Work out the finished part from the listing and answer in its coordinate system (mm). Face numbers are marked on the shaded views. A direction names the side the tool comes from. Round coordinates to 2 decimals unless told otherwise and drop trailing zeros. Write each loop counter-clockwise with the first axis right and the second up, starting at its lowest first coordinate (ties: lowest second). Pieces come first, ordered by that corner, then holes. Notation, with made-up numbers: M 89.25,-16 L 126.25,-16 A32 cw 126.25,23 Z; hole C 26.25,19 d1. An arc over 180 degrees is marked long. One line per item, written item: value. Start each with the question number.
Q1. Find section A-A (y = 0). Write down the section's boundary in (x, z), and give its area (3 significant figures).
Q2. Find section B-B (x = 1). Write down the section's boundary in (y, z), and give its area (3 significant figures).
Q3. Given pin 1 Ø1 at (x, y) = (0, -16.5) entering from +Z; pin 2 Ø2.5 at (x, z) = (-18.5, 1.5) entering from -Y; pin 3 Ø5 at (x, y) = (-19.5, -1) entering from +Z, each flat-ended and moving along its own axis, determine where each tip first touches the part or whether it passes through.
Q4. The mould has two halves that part along X. Classify the marked faces 1, 2 and 3: released by +X, released by -X, zero draft, split by the parting line, or undercut.
Q5. Consider probe 1 along X at (y, z) = (12, 6.75); probe 2 along X at (y, z) = (12, 8.5); probe 3 along Y at (x, z) = (-9, 13.75). Determine where each line is inside the solid, lowest interval first.
Q6. Find section C-C (z = 6). Write down the section's boundary in (x, y).
Q7. Find section D-D (z = 11.25). Write down the section's boundary in (x, y), and give its area (3 significant figures).
Q8. A tool of negligible diameter and unlimited length cuts with its end or side. For the marked faces 4, 5 and 6, from which of +Z, -Z, +X, -X, +Y, -Y can it reach the whole face along a straight path? Write none if from no direction.
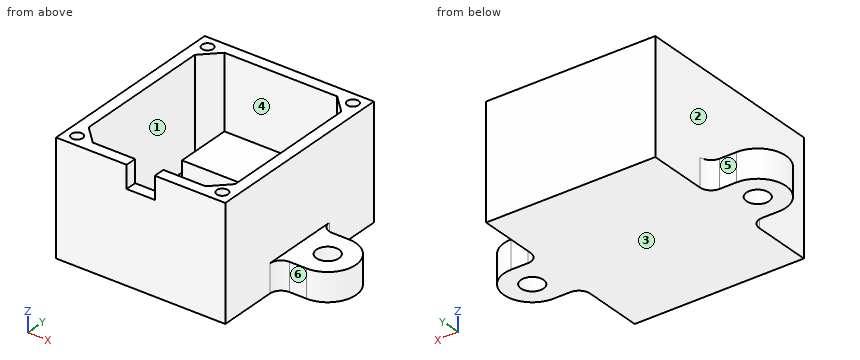
from build123d import *

# Parameters (mm, degrees)
ESQUISSE1_W             = 30
ESQUISSE1_H             = 35
BOSS_EXTRU_1_DEPTH      = 20
ENL_V_MAT_EXTRU_1_DEPTH = 18
BOSS_EXTRU_2_DEPTH      = 5
ENL_V_MAT_EXTRU_2_REACH = 7
ESQUISSE4_R             = 2
ESQUISSE5_W             = 20
ESQUISSE5_H             = 10
BOSS_EXTRU_3_DEPTH      = 5
ENL_V_MAT_EXTRU_3_REACH = 37
ESQUISSE6_W             = 5
ESQUISSE6_H             = 4
CONG_1_R                = 2
ESQUISSE7_R             = 1
ENL_V_MAT_EXTRU_4_DEPTH = 10


with BuildPart() as part:
    # Esquisse1 → Boss.-Extru.1 (new body)
    with BuildSketch(Plane.XY):
        Rectangle(ESQUISSE1_W, ESQUISSE1_H)
    extrude(amount=BOSS_EXTRU_1_DEPTH)

    # Esquisse2 → Enlèv. mat.-Extru.1 (cut)
    with BuildSketch(Plane.XY.offset(20)):
        Polygon((-10, 15.5), (10, 15.5), (13, 12.5), (13, -12.5), (10, -15.5), (-10, -15.5), (-13, -12.5), (-13, 12.5), align=None)
    extrude(amount=-ENL_V_MAT_EXTRU_1_DEPTH, mode=Mode.SUBTRACT)

    # Esquisse3 → Boss.-Extru.2 (add)
    with BuildSketch(Plane(origin=(0, 0, 0), x_dir=(-1, 0, 0), z_dir=(0, 0, -1))):
        with BuildLine():
            Line((-15, 5), (-20, 5))
            ThreePointArc((-20, 5), (-25, 0), (-20, -5))
            Line((-20, -5), (-15, -5))
            Line((-15, -5), (-15, 5))
        make_face()
        with BuildLine():
            Line((15, 5), (15, -5))
            Line((15, -5), (20, -5))
            ThreePointArc((20, -5), (25, 0), (20, 5))
            Line((20, 5), (15, 5))
        make_face()
    extrude(amount=-BOSS_EXTRU_2_DEPTH)

    # Esquisse4 → Enlèv. mat.-Extru.2 (cut, up to next)
    with BuildSketch(Plane.XY.offset(5), mode=Mode.PRIVATE) as enl_v_mat_extru_2_sk1:
        with Locations((-20, 0)):
            Circle(ESQUISSE4_R)
    enl_v_mat_extru_2_tool1 = extrude(enl_v_mat_extru_2_sk1.sketch, amount=-ENL_V_MAT_EXTRU_2_REACH, mode=Mode.PRIVATE) & part.part
    add(enl_v_mat_extru_2_tool1.solids().sort_by_distance((-20, 0, 5))[0], mode=Mode.SUBTRACT)
    # Esquisse4 → Enlèv. mat.-Extru.2 (cut, up to next)
    with BuildSketch(Plane.XY.offset(5), mode=Mode.PRIVATE) as enl_v_mat_extru_2_sk2:
        with Locations((20, 0)):
            Circle(ESQUISSE4_R)
    enl_v_mat_extru_2_tool2 = extrude(enl_v_mat_extru_2_sk2.sketch, amount=-ENL_V_MAT_EXTRU_2_REACH, mode=Mode.PRIVATE) & part.part
    add(enl_v_mat_extru_2_tool2.solids().sort_by_distance((20, 0, 5))[0], mode=Mode.SUBTRACT)

    # Esquisse5 → Boss.-Extru.3 (add)
    with BuildSketch(Plane.XY.offset(2)):
        with Locations((0, 10.5)):
            Rectangle(ESQUISSE5_W, ESQUISSE5_H)
    extrude(amount=BOSS_EXTRU_3_DEPTH)

    # Esquisse6 → Enlèv. mat.-Extru.3 (cut, up to next)
    with BuildSketch(Plane.XZ.offset(17.5), mode=Mode.PRIVATE) as enl_v_mat_extru_3_sk1:
        with Locations((0, 18)):
            Rectangle(ESQUISSE6_W, ESQUISSE6_H)
    enl_v_mat_extru_3_tool1 = extrude(enl_v_mat_extru_3_sk1.sketch, amount=-ENL_V_MAT_EXTRU_3_REACH, mode=Mode.PRIVATE) & part.part
    add(enl_v_mat_extru_3_tool1.solids().sort_by_distance((0, -17.5, 18))[0], mode=Mode.SUBTRACT)

    # Congé1
    cong_1_edges = [part.edges().sort_by_distance(p)[0] for p in [
        (15, -5, 2.5),
        (15, 5, 2.5),
        (-15, 5, 2.5),
        (-15, -5, 2.5),
    ]]
    fillet(cong_1_edges, radius=CONG_1_R)

    # Esquisse7 → Enlèv. mat.-Extru.4 (cut)
    with BuildSketch(Plane.XY.offset(20)):
        with Locations((-12.878679656, 15.378679656)):
            Circle(ESQUISSE7_R)
        with Locations((-12.878679656, -15.378679656)):
            Circle(ESQUISSE7_R)
        with Locations((12.878679656, -15.378679656)):
            Circle(ESQUISSE7_R)
        with Locations((12.878679656, 15.378679656)):
            Circle(ESQUISSE7_R)
    extrude(amount=-ENL_V_MAT_EXTRU_4_DEPTH, mode=Mode.SUBTRACT)


solid = part.part
The answers:
1. outline: M -25,0 L -22,0 L -22,5 L -25,5 Z; M -18,0 L 18,0 L 18,5 L 15,5 L 15,20 L 13,20 L 13,2 L -13,2 L -13,20 L -15,20 L -15,5 L -18,5 Z; M 22,0 L 25,0 L 25,5 L 22,5 Z
1. area: 192 mm2
2. outline: M -17.5,0 L 17.5,0 L 17.5,20 L 15.5,20 L 15.5,7 L 5.5,7 L 5.5,2 L -15.5,2 L -15.5,16 L -17.5,16 Z
2. area: 184 mm2
3. pin 1: z = 16
3. pin 2: y = -5
3. pin 3: z = 5
4. face 1: undercut
4. face 2: released by -X
4. face 3: zero draft
5. probe 1: -15 to -13, -10 to 10, 13 to 15
5. probe 2: -15 to -13, 13 to 15
5. probe 3: -17.5 to -15.5, 15.5 to 17.5
6. outline: M -15,-17.5 L 15,-17.5 L 15,17.5 L -15,17.5 Z; hole M -13,-12.5 L -10,-15.5 L 10,-15.5 L 13,-12.5 L 13,12.5 L 10,15.5 L 10,5.5 L -10,5.5 L -10,15.5 L -13,12.5 Z
7. outline: M -15,-17.5 L 15,-17.5 L 15,17.5 L -15,17.5 Z; hole C -12.88,-15.38 d2; hole C -12.88,15.38 d2; hole M -13,-12.5 L -10,-15.5 L 10,-15.5 L 13,-12.5 L 13,12.5 L 10,15.5 L -10,15.5 L -13,12.5 Z; hole C 12.88,-15.38 d2; hole C 12.88,15.38 d2
7. area: 249 mm2
8. face 4: +Z
8. face 5: +Z, -Z, -X, +Y
8. face 6: +Z, -Z, +X, -Y
